Build history of the part. All positions in model axes, mm. A direction names the side the tool comes from. Give positions to 0.01 mm unless a question says otherwise; leave off trailing zeros. Loops run counter-clockwise (first coordinate to the right, second up) from the corner with the lowest first, then second, coordinate; pieces in that order, holes last. Notation, with made-up numbers: (88, 22.5) -> (136, 22.5) arc R24 ccw to (136, 60.5) -> close; hole circle Ø8 at (-28.5, -39). An arc over 180 degrees is marked (long way). Answer as a JSON object with one key per item and string values. Group by question number.
Q1. Band-saw the part on B-B, the plane z = 4.5. Write the cut outline in (x, y), plus the area to 3 significant figures.
Q2. Band-saw the part on D-D, the plane z = 10.75. Write the cut outline in (x, y), plus the area to 3 significant figures.
Q3. Wall check: probe 1 along X at (y, z) = (38.5, 12); probe 2 along X at (y, z) = (21, 12); probe 3 along Y at (x, z) = (0, 1.45). Give the ranges that are in metal, low to high. Write a range as from..to.
Q4. Drop flat-ended pins along their axis: pin 1 (5 mm diameter, centred on x = 7.5, y = 38, fed in from -Z); pin 2 (7 mm diameter, centred on x = -3, z = 20, fed in from +Y); pin 3 (3.5 mm diameter, centred on x = 0, y = 10, fed in from +Z); pin 4 (6 mm diameter, centred on x = 0.5, y = 14, fed in from +Z). Give the stop position or say it passes through.
Q5. Two-plate mould, pull along Z, no slides. Class faces 1 (the cylindrical face through (0.78, 40.24, 14.48)), 2 (the flat face through (0, 40, 22)), 3 (the flat face through (3, 8.2, 4.9)): pulls with the +Z half, pulls with the -Z half, needs draft (parallel to the pull), parting line crosses it, or undercut.
Q6. Tool access for faces 4 (the flat face through (-6, 23, 12)), 5 (the flat face through (0, 43, 19)), 6 (the flat face through (10, 27, 8)), 7 (the flat face through (0, 43, 4)), 8 (the flat face through (2, 12, 3.2)): list every direction of +Z, -Z, +X, -X, +Y, -Y with a clear straight run to the whole face (end or side of a thin tool).
Q7. Band-saw the part on A-A, the plane x = 0. Write the cut outline in (y, z), plus the area to 3 significant figures.
Q8. Band-saw the part on C-C, the plane y = 40. Write the cut outline in (x, z), plus the area to 3 significant figures.
from build123d import *

# Parameters (mm, degrees)
SKETCH_3_W          = 20
SKETCH_3_H          = 37
EXTRUDE_2_DEPTH     = 6.6
SKETCH_10_R         = 2.2
CUT_EXTRUDE_3_DEPTH = 39.891644347
CUT_EXTRUDE_2_DEPTH = 3.4
SKETCH_11_W         = 20
SKETCH_11_H         = 22
EXTRUDE_5_DEPTH     = 6
SKETCH_9_W          = 20
SKETCH_9_H          = 7.4
EXTRUDE_4_DEPTH     = 0.4
SKETCH_13_R         = 2.6
CUT_EXTRUDE_4_DEPTH = 50.674540763
EXTRUDE_6_DEPTH     = 4


with BuildPart() as part:
    # Эскиз3 → Бобышка-Вытянуть2 (new body)
    with BuildSketch(Plane.XY):
        with Locations((0, 18.5)):
            Rectangle(SKETCH_3_W, SKETCH_3_H)
    extrude(amount=EXTRUDE_2_DEPTH)

    # Эскиз10 → Вырез-Вытянуть3 (cut, through all)
    with BuildSketch(Plane(origin=(0, 0, 0), x_dir=(-1, 0, 0), z_dir=(0, 0, -1))):
        with Locations((0, 10)):
            Circle(SKETCH_10_R)
    extrude(amount=-CUT_EXTRUDE_3_DEPTH, mode=Mode.SUBTRACT)

    # Эскиз6 → Вырез-Вытянуть2 (cut)
    with BuildSketch(Plane.XY.offset(6.6)):
        Polygon((4.041451884, 10), (2.020725942, 13.5), (-2.020725942, 13.5), (-4.041451884, 10), (-2.020725942, 6.5), (2.020725942, 6.5), align=None)
    extrude(amount=-CUT_EXTRUDE_2_DEPTH, mode=Mode.SUBTRACT)

    # Эскиз11 → Бобышка-Вытянуть5 (add)
    with BuildSketch(Plane(origin=(0, 37, 0), x_dir=(1, 0, 0), z_dir=(0, 1, 0))):
        with Locations((0, -11)):
            Rectangle(SKETCH_11_W, SKETCH_11_H)
    extrude(amount=EXTRUDE_5_DEPTH)

    # Эскиз9 → Бобышка-Вытянуть4 (add)
    with BuildSketch(Plane(origin=(0, 43, -43.4), x_dir=(1, 0, 0), z_dir=(0, -1, 0))):
        with Locations((0, 55.4)):
            Rectangle(SKETCH_9_W, SKETCH_9_H)
    extrude(amount=-EXTRUDE_4_DEPTH)

    # Эскиз13 → Вырез-Вытянуть4 (cut, through all)
    with BuildSketch(Plane(origin=(0, 43.4, 0), x_dir=(1, 0, 0), z_dir=(0, 1, 0))):
        with Locations(Location((0, -12, 0), (0, 0, 270))):
            Circle(SKETCH_13_R)
    extrude(amount=-CUT_EXTRUDE_4_DEPTH, mode=Mode.SUBTRACT)

    # Эскиз17 → Бобышка-Вытянуть6 (add)
    with BuildSketch(Plane.ZY.offset(10)):
        Polygon((22, 37), (6.6, 37), (6.6, 0), align=None)
    extrude_6 = extrude(amount=-EXTRUDE_6_DEPTH)

    # Зеркальное отражение1: Бобышка-Вытянуть6 across plane
    add(extrude_6.mirror(Plane(origin=(0, 0, 0), x_dir=(0, 0, 1), z_dir=(1, 0, 0))))


solid = part.part
Worked answers:
{
 "1": {"outline": "(-10, 0) -> (10, 0) -> (10, 43) -> (-10, 43) -> close; hole (-4.04, 10) -> (-2.02, 6.5) -> (2.02, 6.5) -> (4.04, 10) -> (2.02, 13.5) -> (-2.02, 13.5) -> close", "area": "818 mm2"},
 "2": {"outline": "(-10, 9.97) -> (-6, 9.97) -> (-6, 37) -> (-2.28, 37) -> (-2.28, 43.4) -> (-10, 43.4) -> close; (2.28, 37) -> (6, 37) -> (6, 9.97) -> (10, 9.97) -> (10, 43.4) -> (2.28, 43.4) -> close", "area": "315 mm2"},
 "3": {"probe 1": "-10..-2.6, 2.6..10", "probe 2": "-10..-6, 6..10", "probe 3": "0..7.8, 12.2..43"},
 "4": {"pin 1": "z = 0", "pin 2": "y = 43", "pin 3": "through", "pin 4": "z = 6.6"},
 "5": {"face 1": "undercut", "face 2": "pulls with the +Z half", "face 3": "needs draft"},
 "6": {"face 4": "+Z, -Y", "face 5": "+Z, +X, -X, +Y", "face 6": "+Z, -Z, +X, +Y, -Y", "face 7": "-Z, +X, -X, +Y", "face 8": "+Z"},
 "7": {"outline": "(0, 0) -> (7.8, 0) -> (7.8, 3.2) -> (6.5, 3.2) -> (6.5, 6.6) -> (0, 6.6) -> close; (12.2, 0) -> (43, 0) -> (43, 8.3) -> (43.4, 8.3) -> (43.4, 9.4) -> (37, 9.4) -> (37, 6.6) -> (13.5, 6.6) -> (13.5, 3.2) -> (12.2, 3.2) -> close; (37, 14.6) -> (43.4, 14.6) -> (43.4, 15.7) -> (43, 15.7) -> (43, 22) -> (37, 22) -> close", "area": "308 mm2"},
 "8": {"outline": "(-10, 0) -> (10, 0) -> (10, 22) -> (-10, 22) -> close; hole circle Ø5.2 at (0, 12)", "area": "419 mm2"}
}
